from build123d import *

# Parameters (mm, degrees)
F2_R     = 10.7
F2_R_2   = 8.7
F3_DEPTH = 4.5
F5_DEPTH = 10.701
F6_DEPTH = 0.5


with BuildPart() as f3:
    # F2 (on Front) → F3 (new body)
    with BuildSketch(Plane.XZ):
        Circle(F2_R)
        Circle(F2_R_2, mode=Mode.SUBTRACT)
    extrude(amount=F3_DEPTH)

    # F4 (on Top) → F5 (cut, through all)
    with BuildSketch(Plane.XY):
        with BuildLine():
            Line((1.85, -4.5), (1.85, -2.35))
            ThreePointArc((1.85, -2.35), (0, -0.5), (-1.85, -2.35))
            Line((-1.85, -2.35), (-1.85, -4.5))
            Line((-1.85, -4.5), (1.85, -4.5))
        make_face()
    extrude(amount=-F5_DEPTH, mode=Mode.SUBTRACT)

    # F2 (on Front) → F6 (join)
    with BuildSketch(Plane.XZ):
        Circle(F2_R_2)
    extrude(amount=F6_DEPTH)


solid = f3.part
CAD build for the part. Positions are in the model's coordinates, mm. A direction names the side the tool comes from. Round coordinates to 2 decimals unless told otherwise and drop trailing zeros. Loops run counter-clockwise (first coordinate to the right, second up) from the corner with the lowest first, then second, coordinate; pieces in that order, holes last.
(1) Two-plate mould, pull along Z, no slides. Class faces 3 (the flat face through (-1.85, -3, -10)), 4 (the cylindrical face through (-2.32, -2.218, -10.446)), 5 (the flat face through (0, -0.5, 0)): +Z half, -Z half, draft (parallel to the pull), parting line (faces both ways), or undercut.
(2) Which spindle directions (+Z, -Z, +X, -X, +Y, -Y) get a long thin tool onto all of the face, cutting with end or side? Do faces 1 (the flat face through (1.85, -3, -10)), 2 (the flat face through (1, -4.5, 9)). Say none if no direction does.
(3) Wall check: line 1 along X through (y, z) = (-1.85, 0); line 2 along Y through (x, z) = (0.25, -4.5); line 3 along X through (y, z) = (-3.8, 5.5). Give the ranges that are in metal, low to high.
(4) Cut at C-C (y = -4.1). Give the cut face in (x, z), plus the area to 3 significant figures.
(5) Cut at D-D (y = -1.4). Give the cut face in (x, z).
(6) Drop flat-ended pins along their axis: pin 1 (2 mm diameter, centred on y = -4, z = -9.5, fed in from -X); pin 2 (0.6 mm diameter, centred on y = -3.5, z = -10, fed in from +X). Give the stop position or say it passes through.
(7) Cut at A-A (z = 0.5). Give the cut face in (x, y).
(8) Cut at B-B (x = 8). Give the cut face in (y, z).
Findings below:
1. face 3: draft
1. face 4: parting line
1. face 5: undercut
2. face 1: -Z, -Y
2. face 2: +Z, -Z, +X, -X, -Y
3. line 1: x = -10.7 to -8.7, 8.7 to 10.7
3. line 2: y = -0.5 to 0
3. line 3: x = -9.18 to -6.74, 6.74 to 9.18
4. outline: (-1.85, -10.54) - (-1.85, -8.5) arc R8.7 cw (long way) to (1.85, -8.5) - (1.85, -10.54) arc R10.7 ccw (long way) to start
4. area: 114 mm2
5. outline: (-1.59, -10.58) - (-1.59, -8.55) arc R8.7 cw (long way) to (1.59, -8.55) - (1.59, -10.58) arc R10.7 ccw (long way) to start
6. pin 1: stops at x = -6.5
6. pin 2: stops at x = 4.52
7. outline: (-10.69, -4.5) - (-8.69, -4.5) - (-8.69, -0.5) - (8.69, -0.5) - (8.69, -4.5) - (10.69, -4.5) - (10.69, 0) - (-10.69, 0) - close
8. outline: (-4.5, -7.11) - (0, -7.11) - (0, 7.11) - (-4.5, 7.11) - (-4.5, 3.42) - (-0.5, 3.42) - (-0.5, -3.42) - (-4.5, -3.42) - close
